from build123d import *

# Parameters (mm, degrees)
SKETCH1_W                    = 76.2
SKETCH1_H                    = 50.038
SKETCH1_R                    = 7.9375
BASE_FLANGE1_DEPTH           = 1.27
EDGE_FLANGE1_STRIP_W         = 7.62
EDGE_FLANGE1_STRIP_H         = 1.27
EDGE_FLANGE1_STRIP_CUT_DEPTH = 76.2
EDGE_FLANGE1_DEPTH           = 76.2
SKETCH9_R                    = 1.651
CUT_EXTRUDE3_DEPTH           = 52.076899093
CIRPATTERN2_COUNT            = 4
SKETCH11_R                   = 6.35
SKETCH11_R_2                 = 1.651
CUT_EXTRUDE4_DEPTH           = 2.54
CIRPATTERN3_COUNT            = 4
CUT_EXTRUDE2_DEPTH           = 69.426487445
CUT_EXTRUDE2_DEPTH_BACK      = 69.426487445
SKETCH10_R                   = 1.5875


# Sheet-metal steps are written as plain solids
with BuildPart() as part:
    # Sketch1 → Base-Flange1 (new body)
    with BuildSketch(Plane(origin=(0, 0, 0), x_dir=(1, 0, 0), z_dir=(0, 1, 0))):
        Rectangle(SKETCH1_W, SKETCH1_H)
        with Locations(Location((-19.05, 0, 0), (0, 0, 270))):
            Circle(SKETCH1_R, mode=Mode.SUBTRACT)
    extrude(amount=-BASE_FLANGE1_DEPTH)

    # Edge-Flange1 strip (across the edge) → Edge-Flange1 strip cut (cut)
    with BuildSketch(Plane(origin=(-38.1, 0, 25.019), x_dir=(0, 0, -1), z_dir=(1, 0, 0))):
        with Locations((-2.54, -0.635)):
            Rectangle(EDGE_FLANGE1_STRIP_W, EDGE_FLANGE1_STRIP_H)
    edge_flange1_strip_cut = extrude(amount=EDGE_FLANGE1_STRIP_CUT_DEPTH, mode=Mode.SUBTRACT)

    # Edge-Flange1 section (across the edge) → Edge-Flange1 (add)
    with BuildSketch(Plane(origin=(-38.1, 0, 25.019), x_dir=(0, 0, -1), z_dir=(1, 0, 0))):
        with BuildLine():
            Line((-1.27, 1.27), (-1.27, 21.59))
            Line((-1.27, 21.59), (0, 21.59))
            Line((0, 21.59), (0, 1.27))
            ThreePointArc((0, 1.27), (0.371974388, 0.371974388), (1.27, 0))
            Line((1.27, 0), (1.27, -1.27))
            ThreePointArc((1.27, -1.27), (-0.526051224, -0.526051224), (-1.27, 1.27))
        make_face()
    edge_flange1 = extrude(amount=EDGE_FLANGE1_DEPTH)

    # Mirror1: Edge-Flange1 strip cut, Edge-Flange1 across plane
    add(edge_flange1_strip_cut.mirror(Plane.XY), mode=Mode.SUBTRACT)
    add(edge_flange1.mirror(Plane.XY))

    # Sketch9 → Cut-Extrude3 (cut, through all)
    with BuildSketch(Plane(origin=(0, 0, 0), x_dir=(1, 0, 0), z_dir=(0, 1, 0))):
        with Locations(Location((-32.520384182, 13.470384182, 0), (0, 0, 270))):
            Circle(SKETCH9_R)
    cut_extrude3 = extrude(amount=-CUT_EXTRUDE3_DEPTH, mode=Mode.SUBTRACT)

    # CirPattern2: Cut-Extrude3 ×4 about axis
    cirpattern2_axis = Axis((-19.05, 0, 0), (0, 1, 0))
    for i in range(1, CIRPATTERN2_COUNT):
        add(cut_extrude3.rotate(cirpattern2_axis, i * 360 / CIRPATTERN2_COUNT), mode=Mode.SUBTRACT)

    # Sketch11 → Cut-Extrude4 (cut)
    with BuildSketch(Plane(origin=(0, 0, 0), x_dir=(1, 0, 0), z_dir=(0, 1, 0))):
        with Locations(Location((19.05, 0, 0), (0, 0, 270))):
            Circle(SKETCH11_R)
        with Locations(Location((5.579615818, 13.470384182, 0), (0, 0, 270))):
            Circle(SKETCH11_R_2)
    cut_extrude4 = extrude(amount=-CUT_EXTRUDE4_DEPTH, mode=Mode.SUBTRACT)

    # CirPattern3: Cut-Extrude4 ×4 about axis
    cirpattern3_axis = Axis((19.05, 0, 0), (0, 1, 0))
    for i in range(1, CIRPATTERN3_COUNT):
        add(cut_extrude4.rotate(cirpattern3_axis, i * 360 / CIRPATTERN3_COUNT), mode=Mode.SUBTRACT)

    # Sketch10 → Cut-Extrude2 (cut, two sides: drawn at the far end of the back side and taken through both)
    with BuildSketch(Plane(origin=(0, 0, -26.289), x_dir=(-1, 0, 0), z_dir=(0, 0, -1)).offset(-CUT_EXTRUDE2_DEPTH_BACK)):
        with Locations((7.52856, 6.35)):
            Circle(SKETCH10_R)
        with Locations((32.92856, 6.35)):
            Circle(SKETCH10_R)
    extrude(amount=CUT_EXTRUDE2_DEPTH + CUT_EXTRUDE2_DEPTH_BACK, mode=Mode.SUBTRACT)


solid = part.part
The listing builds one solid part. Answer for the finished solid, in the listing's coordinates (mm). A direction names the side the tool comes from. Coordinates: 2 decimals unless noted, no trailing zeros. Loops run counter-clockwise (first coordinate to the right, second up) from the corner with the lowest first, then second, coordinate; pieces in that order, holes last.
1) Find section C-C on z = 0. Write down the section's boundary in (x, y).
2) Find section A-A on y = 6.35. Write down the section's boundary in (x, z).
3) Find the intervals of material crossed by L1, parallel to X at y = -0.25, z = 0; L2, parallel to X at y = 6.35, z = 25.6; L3, parallel to Z at x = -14, y = 6.25, in increasing order.
4) Find section B-B on x = 19.05. Write down the section's boundary in (y, z), then the cut area to 3 significant figures.
5) A tool of negligible diameter and unlimited length cuts with its end or side. For faces 1 (the face through (25.346, -0.626, -0.827)), 2 (the face through (-1, 0, 0)), from which of +Z, -Z, +X, -X, +Y, -Y can it reach the whole face along a straight path? Write none if from no direction.
6) Find section D-D on y = 16.25. Write down the section's boundary in (x, z).
7) Flat-ended cylindrical pins translate along their axes: pin 1 Ø4.5 at (x, z) = (32.52, 13.47) entering from +Y; pin 2 Ø2.5 at (x, y) = (-7.53, 6.35) entering from -Z. Find the tip coordinate at first contact, or state that the pin passes through.
8) Determine the mould class of faces 3 (the face through (-6.27, 5.38, -25.65)), 4 (the face through (38.1, -1, 0)), 5 (the face through (-1, 11, 26.289)) for opening direction X: pulls with the +X half, pulls with the -X half, needs draft (parallel to the pull), parting line crosses it, or undercut.
Values:
1. outline: (-38.1, -1.27) - (-26.99, -1.27) - (-26.99, 0) - (-38.1, 0) - close; (-11.11, -1.27) - (12.7, -1.27) - (12.7, 0) - (-11.11, 0) - close; (25.4, -1.27) - (38.1, -1.27) - (38.1, 0) - (25.4, 0) - close
2. outline: (-38.1, -26.29) - (-34.52, -26.29) - (-34.52, -25.02) - (-38.1, -25.02) - close; (-38.1, 25.02) - (-34.52, 25.02) - (-34.52, 26.29) - (-38.1, 26.29) - close; (-31.34, -26.29) - (-9.12, -26.29) - (-9.12, -25.02) - (-31.34, -25.02) - close; (-31.34, 25.02) - (-9.12, 25.02) - (-9.12, 26.29) - (-31.34, 26.29) - close; (-5.94, -26.29) - (38.1, -26.29) - (38.1, -25.02) - (-5.94, -25.02) - close; (-5.94, 25.02) - (38.1, 25.02) - (38.1, 26.29) - (-5.94, 26.29) - close
3. L1: x = -38.1 to -26.99, -11.11 to 12.7, 25.4 to 38.1
3. L2: x = -38.1 to -34.52, -31.34 to -9.12, -5.94 to 38.1
3. L3: z = -26.29 to -25.02, 25.02 to 26.29
4. outline: (-1.27, -23.75) arc R2.54 ccw to (1.27, -26.29) - (21.59, -26.29) - (21.59, -25.02) - (1.27, -25.02) arc R1.27 cw to (0, -23.75) - (0, -6.35) - (-1.27, -6.35) - close; (-1.27, 6.35) - (0, 6.35) - (0, 23.75) arc R1.27 cw to (1.27, 25.02) - (21.59, 25.02) - (21.59, 26.29) - (1.27, 26.29) arc R2.54 ccw to (-1.27, 23.75) - close
4. area: 103 mm2
5. face 1: +Y, -Y
5. face 2: +X, -X, +Y
6. outline: (-38.1, -26.29) - (38.1, -26.29) - (38.1, -25.02) - (-38.1, -25.02) - close; (-38.1, 25.02) - (38.1, 25.02) - (38.1, 26.29) - (-38.1, 26.29) - close
7. pin 1: stops at y = 0
7. pin 2: passes through
8. face 3: undercut
8. face 4: pulls with the +X half
8. face 5: needs draft
